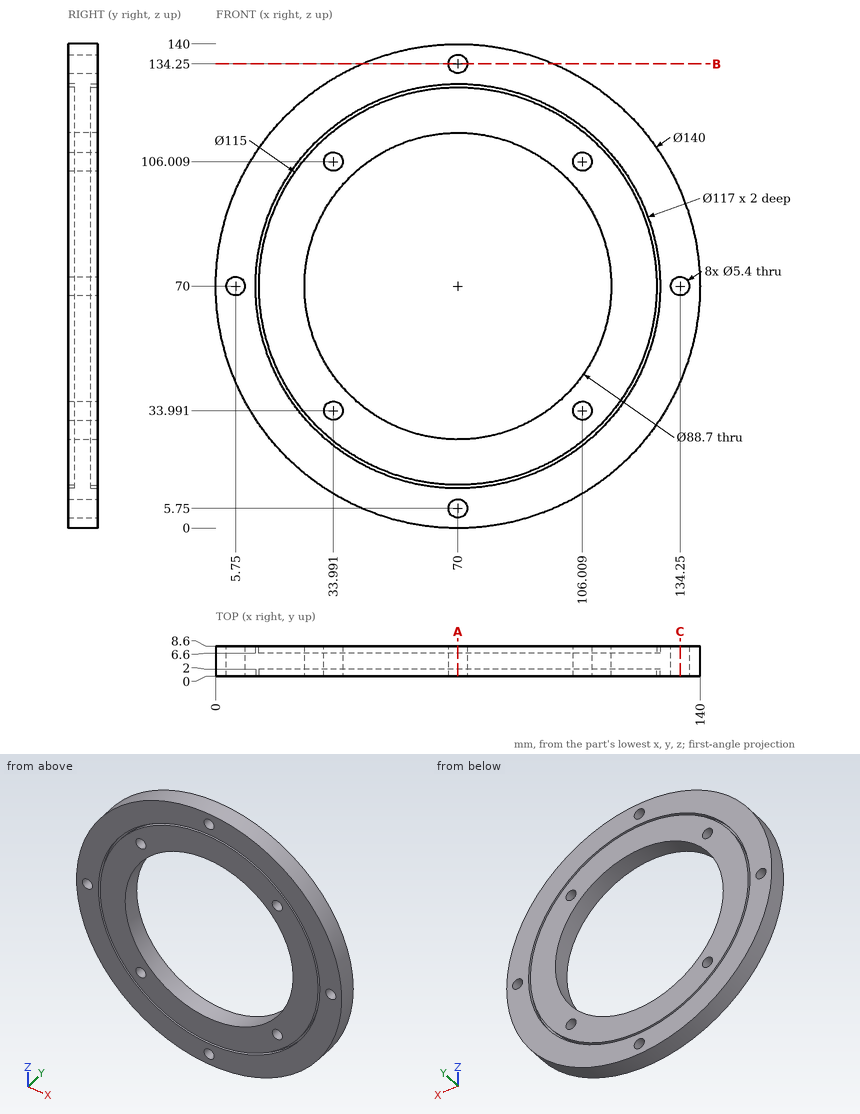
For this review, use the dimensioned drawing (mm, ordinates from the lowest corner) and the shaded views. Give positions to 0.01 mm unless a question says otherwise; leave off trailing zeros. Order: outer loops, then holes, each group sorted by start corner. A loop starts at its lowest first (then second) coordinate and runs counter-clockwise, first axis right, second up. Notation, with made-up numbers: (20, -28.75) - (67, -28.75) arc R5 ccw to (67, -22.75) - close; hole circle Ø9 at (50.25, 54.5). An arc over 180 degrees is marked (long way). Use a Markdown table: item, result. Add a question column.
(1) Wall thickness on probe 1 along Z at (x, y) = (70, 7.55); probe 2 along X at (y, z) = (1.5, 114.5) (1 decimal); probe 3 along X at (y, z) = (5.5, 33.5) (1 decimal): over which ranges is each line inside the solid? List them lowest first. Write a range as [from, to].
(2) Add section A-A on x = 70. Give the number of separate pieces and of enclosed holes in the cut face, then the cut area to 3 significant figures.
(3) Clearance check with flat-ended pins moving along their axes: P1, Ø5, axis at x = 70, z = 5.75, coming from the -Y side; P2, Ø4, axis at y = 6.5, z = 39, coming from the -X side; P3, Ø4, axis at y = 6.5, z = 112.5, coming from the +X side (1 decimal); P4, Ø1, axis at y = 2, z = 92.5, coming from the -X side. State where each tip first meets the part, or that it passes through.
(4) Add section C-C on x = 134.25. Give the boundary of the cut face in (y, z).
(5) Add section B-B on z = 134.25. Give the boundary of the cut face in (x, y).
Report:
| question | item | result |
|---|---|---|
| 1 | probe 1 | z = [0, 3.05], [8.45, 11.5], [12.5, 25.65], [114.35, 127.5], [128.5, 131.55], [136.95, 140] |
| 1 | probe 2 | x = [16, 32], [33.6, 106.4], [108, 124] |
| 1 | probe 3 | x = [10.3, 31.3], [36.6, 44.8], [95.2, 103.4], [108.7, 129.7] |
| 2 | separate pieces | 4 |
| 2 | enclosed holes | 0 |
| 2 | area | 340 mm² |
| 3 | P1 | passes through |
| 3 | P2 | stops at x = 6.29 |
| 3 | P3 | stops at x = 127.1 |
| 3 | P4 | stops at x = 3.55 |
| 4 | outline | (0, 42.22) - (8.6, 42.22) - (8.6, 67.3) - (0, 67.3) - close; (0, 72.7) - (8.6, 72.7) - (8.6, 97.78) - (0, 97.78) - close |
| 5 | outline | (42.22, 0) - (67.3, 0) - (67.3, 8.6) - (42.22, 8.6) - close; (72.7, 0) - (97.78, 0) - (97.78, 8.6) - (72.7, 8.6) - close |
